Check sheet for the modelled part. Datum: model origin and axes. Units: mm. Face numbers are marked on the shaded views. A direction names the side the tool comes from. Coordinates: 2 decimals unless noted, no trailing zeros. Loops run counter-clockwise (first coordinate to the right, second up) from the corner with the lowest first, then second, coordinate; pieces in that order, holes last.
```python
from build123d import *

# Parameters (mm, degrees)
BOSS_EXTRUDE1_DEPTH  = 28.8
M5_CLEARANCE_HOLE1_D = 5.5
CUT_EXTRUDE1_DEPTH   = 45.9


with BuildPart() as part:
    # Sketch1 → Boss-Extrude1 (new body)
    with BuildSketch(Plane(origin=(0, 0, 0), x_dir=(1, 0, 0), z_dir=(0, 1, 0))):
        with BuildLine():
            Line((-22.45, 0), (-22.45, 50))
            Line((-22.45, 50), (-18.15, 50))
            Line((-18.15, 50), (-18.15, 0))
            ThreePointArc((-18.15, 0), (0, -18.15), (18.15, 0))
            Line((18.15, 0), (18.15, 50))
            Line((18.15, 50), (22.45, 50))
            Line((22.45, 50), (22.45, 0))
            ThreePointArc((22.45, 0), (0, -22.45), (-22.45, 0))
        make_face()
    extrude(amount=BOSS_EXTRUDE1_DEPTH)

    # M5 Clearance Hole1 (through all)
    with Locations(Plane(origin=(22.45, 0, 0), x_dir=(0, 0, -1), z_dir=(1, 0, 0))):
        with Locations((21.17, 14.4), (35.7, 14.4)):
            Hole(M5_CLEARANCE_HOLE1_D / 2)

    # Sketch5 → Cut-Extrude1 (cut, through all)
    with BuildSketch(Plane(origin=(22.45, 0, 0), x_dir=(0, 0, -1), z_dir=(1, 0, 0))):
        with BuildLine():
            Line((50, 0), (50, 14.4))
            ThreePointArc((50, 14.4), (48.714437262, 6.778320395), (45, 0))
            Line((45, 0), (50, 0))
        make_face()
        with BuildLine():
            Line((50, 28.8), (45, 28.8))
            ThreePointArc((45, 28.8), (48.714437262, 22.021679605), (50, 14.4))
            Line((50, 14.4), (50, 28.8))
        make_face()
    extrude(amount=-CUT_EXTRUDE1_DEPTH, mode=Mode.SUBTRACT)


solid = part.part
```
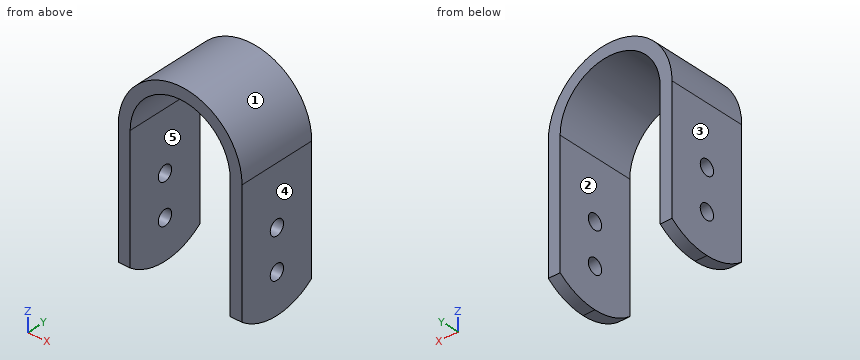
1) Section check D-D on y = 22.25. Enter the section's corners in (x, z), plus the area to 3 significant figures.
Answer sheet:
outline: (-22.45, -48.63) - (-18.15, -48.63) - (-18.15, 0) arc R18.15 cw to (18.15, 0) - (18.15, -48.63) - (22.45, -48.63) - (22.45, 0) arc R22.45 ccw to (-22.45, 0) - close
area: 692 mm2
2) Set-up check for the marked faces 4 and 5: record each of +Z, -Z, +X, -X, +Y, -Y from which the full face is reachable in a straight line by a thin tool's end or side.
Answer sheet:
face 4: +Z, -Z, +X, +Y, -Y
face 5: -Z, +Y, -Y
3) Section check B-B on z = -20. Enter the section's corners in (x, y), plus the area to 3 significant figures.
Answer sheet:
outline: (-22.45, 0) - (-18.15, 0) - (-18.15, 11.91) - (-22.45, 11.91) - close; (-22.45, 16.89) - (-18.15, 16.89) - (-18.15, 28.8) - (-22.45, 28.8) - close; (18.15, 0) - (22.45, 0) - (22.45, 11.91) - (18.15, 11.91) - close; (18.15, 16.89) - (22.45, 16.89) - (22.45, 28.8) - (18.15, 28.8) - close
area: 205 mm2
4) Section check A-A on z = -31.5. Enter the section's corners in (x, y).
Answer sheet:
outline: (-22.45, 0) - (-18.15, 0) - (-18.15, 28.8) - (-22.45, 28.8) - close; (18.15, 0) - (22.45, 0) - (22.45, 28.8) - (18.15, 28.8) - close
5) Scan lines: line 1 (X direction, y = 13.25, z = -5); line 2 (Y direction, x = -20.6, z = -35.7); line 3 (X direction, y = 3.5, z = 8). Record each from-to range of solid material in increasing order.
Answer sheet:
line 1: x = -22.45 to -18.15, 18.15 to 22.45
line 2: y = 0 to 11.65, 17.15 to 28.8
line 3: x = -20.98 to -16.29, 16.29 to 20.98
6) Depth check by flat-ended pin: pin 1 (12 mm diameter, centred on x = -17, y = 19, fed in from +Z); pin 2 (6 mm diameter, centred on x = 17, y = 16.5, fed in from +Z); pin 3 (10 mm diameter, centred on x = 14.5, y = 20.5, fed in from -Z). Enter the tip coordinate at first touch or a pass-through.
Answer sheet:
pin 1: stops at z = 19.57
pin 2: stops at z = 17.55
pin 3: stops at z = -49.84
7) Mould release check, pull along X, two halves, no side actions. Record for the marked faces 1, 2 and 3: +X half, -X half, draft (parallel to the pull), parting line (faces both ways), or undercut.
Answer sheet:
face 1: parting line
face 2: undercut
face 3: -X half
8) Section check C-C on y = 12.5. Enter the section's corners in (x, z).
Answer sheet:
outline: (-22.45, -49.92) - (-18.15, -49.92) - (-18.15, -37.69) - (-22.45, -37.69) - close; (-22.45, -33.71) - (-18.15, -33.71) - (-18.15, -23.16) - (-22.45, -23.16) - close; (-22.45, -19.18) - (-18.15, -19.18) - (-18.15, 0) arc R18.15 cw to (18.15, 0) - (18.15, -19.18) - (22.45, -19.18) - (22.45, 0) arc R22.45 ccw to (-22.45, 0) - close; (18.15, -49.92) - (22.45, -49.92) - (22.45, -37.69) - (18.15, -37.69) - close; (18.15, -33.71) - (22.45, -33.71) - (22.45, -23.16) - (18.15, -23.16) - close
